The figure shows three views and two pictorial views of one solid part (mm, origin at its lowest corner). Answer the questions. A direction names the side the tool comes from. Round coordinates to 2 decimals unless told otherwise and drop trailing zeros. Order: outer loops, then holes, each group sorted by start corner. A loop starts at its lowest first (then second) coordinate and runs counter-clockwise, first axis right, second up. Notation, with made-up numbers: (-35, -30.5) - (-15, -30.5) arc R24 cw to (-15, -18.5) - close; hole circle Ø8 at (-1.5, 27.5). An arc over 180 degrees is marked (long way). Answer in a Markdown table with one row per item.
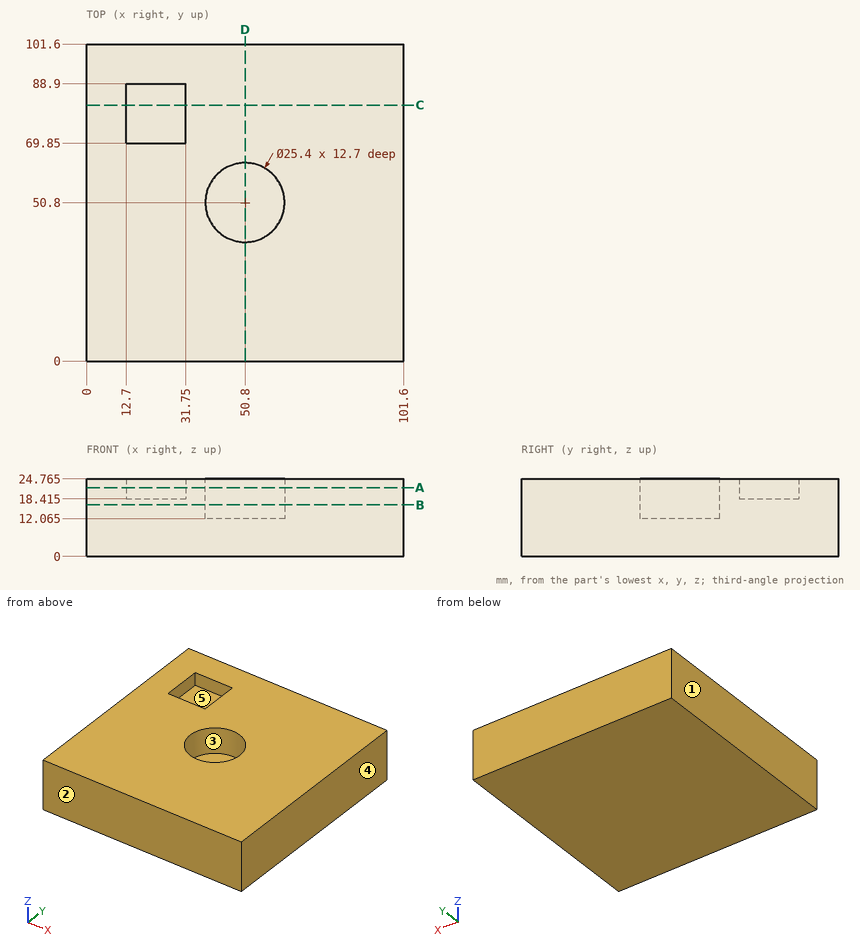
1) Each of these flat-tipped pins is pushed along its axis until it touches: pin 1 (5 mm diameter, centred on x = 25, z = 4.5, fed in from -Y); pin 2 (1.5 mm diameter, centred on x = 59.5, y = 50.5, fed in from +Z) (3 decimals); pin 3 (5.5 mm diameter, centred on x = 26.5, y = 75, fed in from +Z) (3 decimals). Where does it stop, or does it pass through?
Filled in:
| item | result |
|---|---|
| pin 1 | stops at y = 0 |
| pin 2 | stops at z = 12.065 |
| pin 3 | stops at z = 18.415 |
2) Find section B-B, the plane z = 16.5. Give the vertices of the cut face in (x, y).
Filled in:
| item | result |
|---|---|
| outline | (0, 0) - (101.6, 0) - (101.6, 101.6) - (0, 101.6) - close; hole circle Ø25.4 at (50.8, 50.8) |
3) Find section A-A, the plane z = 22. Give the vertices of the cut face in (x, y), then the cut area to 3 significant figures.
Filled in:
| item | result |
|---|---|
| outline | (0, 0) - (101.6, 0) - (101.6, 101.6) - (0, 101.6) - close; hole (12.7, 69.85) - (31.75, 69.85) - (31.75, 88.9) - (12.7, 88.9) - close; hole circle Ø25.4 at (50.8, 50.8) |
| area | 9,450 mm^2 |
4) Find section D-D, the plane x = 50.8. Give the vertices of the cut face in (y, z) (3 decimals), then the cut area to 3 significant figures.
Filled in:
| item | result |
|---|---|
| outline | (0, 0) - (101.6, 0) - (101.6, 24.765) - (63.5, 24.765) - (63.5, 12.065) - (38.1, 12.065) - (38.1, 24.765) - (0, 24.765) - close |
| area | 2,190 mm^2 |
5) Which of the six approach directions +Z, -Z, +X, -X, +Y, -Y give full straight-line access (tool end or side, diameter ignored) to the marked faces 4 and 5?
Filled in:
| item | result |
|---|---|
| face 4 | +Z, -Z, +X, +Y, -Y |
| face 5 | +Z |
6) The mould has two halves that part along Y. Classify the marked faces 1, 2 and 3: released by +Y, released by -Y, zero draft, split by the parting line, or undercut.
Filled in:
| item | result |
|---|---|
| face 1 | zero draft |
| face 2 | released by -Y |
| face 3 | undercut |
7) Find the intervals of material crossed by probe 1 along Y at (x, z) = (50.8, 19); probe 2 along Y at (x, z) = (62, 18.75); probe 3 along X at (y, z) = (58, 20.5), in increasing order. Write a range as from..to.
Filled in:
| item | result |
|---|---|
| probe 1 | y = 0..38.1, 63.5..101.6 |
| probe 2 | y = 0..44.81, 56.79..101.6 |
| probe 3 | x = 0..40.34, 61.26..101.6 |
8) Find section C-C, the plane y = 82. Give the vertices of the cut face in (x, z) (3 decimals), then the cut area to 3 significant figures.
Filled in:
| item | result |
|---|---|
| outline | (0, 0) - (101.6, 0) - (101.6, 24.765) - (31.75, 24.765) - (31.75, 18.415) - (12.7, 18.415) - (12.7, 24.765) - (0, 24.765) - close |
| area | 2,400 mm^2 |
